Job drawing, mm, ordinate dimensions from the low corner. One solid piece. Round coordinates to 2 decimals unless told otherwise and drop trailing zeros. Loops run counter-clockwise (first coordinate to the right, second up) from the corner with the lowest first, then second, coordinate; pieces in that order, holes last. Notation, with made-up numbers: M -12.75,48.25 L 23.25,48.25 A7 ccw 23.25,56.25 Z; hole C -16,24.25 d1. An arc over 180 degrees is marked long. Use one line per item in the form item = value.
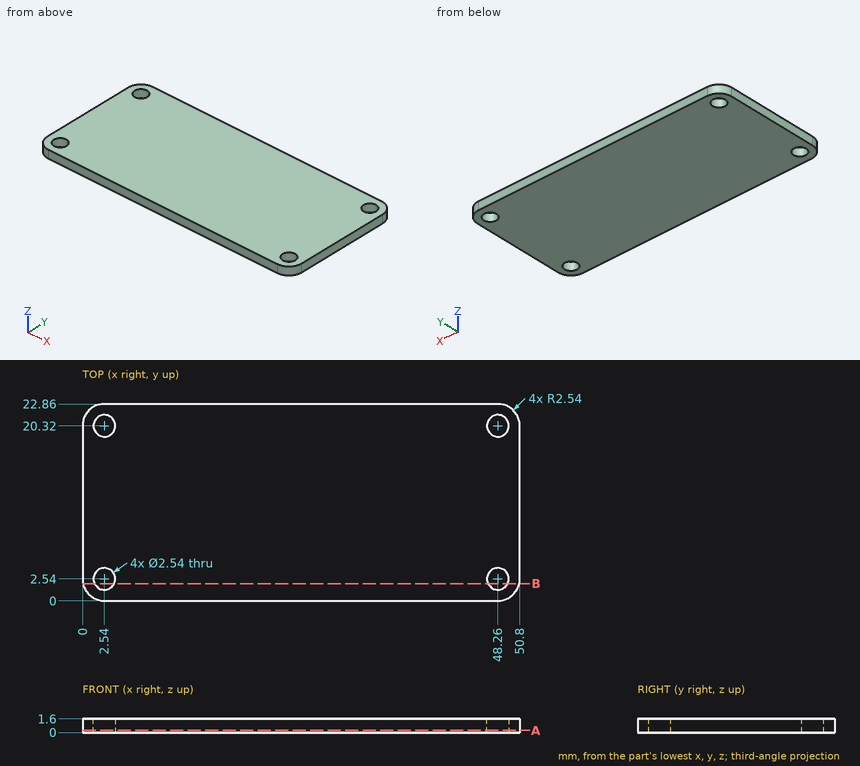
1. Cut at A-A on z = 0.25. Write the cut outline in (x, y), and give its area (3 significant figures).
Completed:
outline = M 0,2.54 A2.54 ccw 2.54,0 L 48.26,0 A2.54 ccw 50.8,2.54 L 50.8,20.32 A2.54 ccw 48.26,22.86 L 2.54,22.86 A2.54 ccw 0,20.32 Z; hole C 2.54,2.54 d2.54; hole C 2.54,20.32 d2.54; hole C 48.26,2.54 d2.54; hole C 48.26,20.32 d2.54
area = 1,140 mm2
2. Probe line 1 along Y through (x, z) = (48.26, 0.3); line 2 along X through (y, z) = (3, 0.75); line 3 along X through (y, z) = (19.25, 1.3). List the from-to ranges inside material, lowest first. Write a range as from..to.
Completed:
line_1 = 0..1.27, 3.81..19.05, 21.59..22.86
line_2 = 0..1.36, 3.72..47.08, 49.44..50.8
line_3 = 0..1.86, 3.22..47.58, 48.94..50.8
3. Drop a flat-ended pin along its axis: P1, Ø3, axis at x = 48.26, y = 2.54, coming from the -Z side. Give the stop position or say it passes through.
Completed:
P1 = 0
4. Cut at B-B on y = 2. Write the cut outline in (x, z).
Completed:
outline = M 0.06,0 L 1.39,0 L 1.39,1.6 L 0.06,1.6 Z; M 3.69,0 L 47.11,0 L 47.11,1.6 L 3.69,1.6 Z; M 49.41,0 L 50.74,0 L 50.74,1.6 L 49.41,1.6 Z
